```python
from build123d import *

# Parameters (mm, degrees)
F0_W     = 1524
F0_H     = 1016
F1_DEPTH = 1016
F2_W     = 254
F2_H     = 508
F3_DEPTH = 1524
F5_DEPTH = 508


with BuildPart() as f1:
    # F0 (on Front) → F1 (new body)
    with BuildSketch(Plane.XZ):
        with Locations((-18.253883, -14.982007)):
            Rectangle(F0_W, F0_H)
    extrude(amount=F1_DEPTH)

    # F2 (on face) → F3 (cut)
    with BuildSketch(Plane.XY.offset(493.017993)):
        with Locations((616.746117, -254)):
            Rectangle(F2_W, F2_H)
    extrude(amount=-F3_DEPTH, mode=Mode.SUBTRACT)

    # F4 (on face) → F5 (cut)
    with BuildSketch(Plane.XZ.offset(1016)):
        Polygon((743.746117, 493.017993), (-780.253883, 493.017993), (-780.253883, -268.982007), (743.746117, -268.982007), (743.746117, 0), (235.746117, 0), (235.746117, 254), (743.746117, 254), align=None)
    extrude(amount=-F5_DEPTH, mode=Mode.SUBTRACT)


solid = f1.part
```
The model under review builds one solid part; all positions refer to its coordinate system, in mm. A direction names the side the tool comes from. Round coordinates to 2 decimals unless told otherwise and drop trailing zeros. Write each loop counter-clockwise with the first axis right and the second up, starting at its lowest first coordinate (ties: lowest second). Pieces come first, ordered by that corner, then holes.
(1) We need section B-B on z = 63. Give the boundary of the cut face in (x, y).
(2) Machinability: for faces 4 (the flat face through (486, -1016, 129)), 5 (the flat face through (486, -766, 254)), 6 (the flat face through (-29, -766, -268.982)), 7 (the flat face through (235.746, -766, 125)), 8 (the flat face through (615, -508, -394)), which of the approach directions +Z, -Z, +X, -X, +Y, -Y give a long, thin tool a straight path to every point of the face, cutting with its end or side? Answer none if there is none.
(3) We need section C-C on x = 312. Give the boundary of the cut face in (y, z), and give its area (3 significant figures).
(4) Insertion check: pin 1 (12 mm diameter, centred on x = -192.5, z = 367, fed in from -Y). The pin has a flat end and moves straight along its axis. Give the tip position at first contact, or say it passes through.
(5) We need section A-A on y = -627. Give the boundary of the cut face in (x, z), and give its area (3 significant figures).
(6) Mouldability with a two-part tool opening along Y and no side actions: class faces 1 (the flat face through (-29, -1016, -394)), 2 (the flat face through (493, -766, 0)), 3 (the flat face through (-154, 0, -8)) as +Y half, -Y half, draft (parallel to the pull), parting line (faces both ways), or undercut.
(7) We need section D-D on y = -398. Give the boundary of the cut face in (x, z), and give its area (3 significant figures).
(8) Wall thickness on L1, parallel to Z at x = 253.5, y = -673; L2, parallel to X at y = -384, z = -159; L3, parallel to Z at x = -371, y = -599: over which ranges is each line inside the solid? List them lowest first.
Findings below:
1. outline: (-780.25, -508) - (235.75, -508) - (235.75, -1016) - (743.75, -1016) - (743.75, -508) - (489.75, -508) - (489.75, 0) - (-780.25, 0) - close
2. face 4: +Z, -Z, +X, -X, -Y
2. face 5: +Z, +X, -X, -Y
2. face 6: +X, -X, -Y
2. face 7: +Z, -X, -Y
2. face 8: +Z, -Z, +X, +Y
3. outline: (-1016, -522.98) - (0, -522.98) - (0, 493.02) - (-508, 493.02) - (-508, 254) - (-1016, 254) - (-1016, 0) - (-508, 0) - (-508, -268.98) - (-1016, -268.98) - close
3. area: 774,000 mm2
4. pin 1: stops at y = -508
5. outline: (-780.25, -522.98) - (743.75, -522.98) - (743.75, -268.98) - (-780.25, -268.98) - close; (235.75, 0) - (743.75, 0) - (743.75, 254) - (235.75, 254) - close
5. area: 516,000 mm2
6. face 1: -Y half
6. face 2: draft
6. face 3: +Y half
7. outline: (-780.25, -522.98) - (489.75, -522.98) - (489.75, 493.02) - (-780.25, 493.02) - close
7. area: 1,290,000 mm2
8. L1: z = -522.98 to -268.98, 0 to 254
8. L2: x = -780.25 to 489.75
8. L3: z = -522.98 to -268.98
